```python
from build123d import *

# Parameters (mm, degrees)
F0_R     = 6.35
F1_DEPTH = 5.08
F2_SIZE  = 5.07999


# Not quite as in the source:
# - a fillet or chamfer is up to 0.001 mm smaller than in the source, because OpenCascade refuses the exact size


with BuildPart() as f1:
    # F0 (on Top) → F1 (new body)
    with BuildSketch(Plane.XY):
        with BuildLine():
            ThreePointArc((-16.2956875, 7.1118892639), (-12.5723585695, 12.5723585695), (-7.1118892639, 16.2956875))
            ThreePointArc((-7.1118892639, 16.2956875), (-6.7408857543, 18.5233780558), (-5.6901704054, 20.5224393535))
            Line((-5.6901704054, 20.5224393535), (-34.321730181, 34.321730181))
            Line((-34.321730181, 34.321730181), (-20.5224393535, 5.6901704054))
            ThreePointArc((-20.5224393535, 5.6901704054), (-18.5233780558, 6.7408857543), (-16.2956875, 7.1118892639))
        make_face()
        with BuildLine():
            ThreePointArc((16.2956875, -7.1118892639), (9.144, 0), (16.2956875, 7.1118892639))
            ThreePointArc((16.2956875, 7.1118892639), (12.5723585695, 12.5723585695), (7.1118892639, 16.2956875))
            ThreePointArc((7.1118892639, 16.2956875), (7.1119723159, 16.2758438272), (7.112, 16.256))
            ThreePointArc((7.112, 16.256), (-0.0198438272, 9.1440276841), (-7.1118892639, 16.2956875))
            ThreePointArc((-7.1118892639, 16.2956875), (-12.5723585695, 12.5723585695), (-16.2956875, 7.1118892639))
            ThreePointArc((-16.2956875, 7.1118892639), (-11.2411078526, 5.042955557), (-9.144, 0))
            ThreePointArc((-9.144, 0), (-11.2411078526, -5.042955557), (-16.2956875, -7.1118892639))
            ThreePointArc((-16.2956875, -7.1118892639), (-12.5723585695, -12.5723585695), (-7.1118892639, -16.2956875))
            ThreePointArc((-7.1118892639, -16.2956875), (-0.0198438272, -9.1440276841), (7.112, -16.256))
            ThreePointArc((7.112, -16.256), (7.1119723159, -16.2758438272), (7.1118892639, -16.2956875))
            ThreePointArc((7.1118892639, -16.2956875), (12.5723585695, -12.5723585695), (16.2956875, -7.1118892639))
        make_face()
        Circle(F0_R, mode=Mode.SUBTRACT)
        with BuildLine():
            ThreePointArc((7.1118892639, 16.2956875), (12.5723585695, 12.5723585695), (16.2956875, 7.1118892639))
            ThreePointArc((16.2956875, 7.1118892639), (18.5233780558, 6.7408857543), (20.5224393535, 5.6901704054))
            Line((20.5224393535, 5.6901704054), (34.321730181, 34.321730181))
            Line((34.321730181, 34.321730181), (5.6901704054, 20.5224393535))
            ThreePointArc((5.6901704054, 20.5224393535), (6.7408857543, 18.5233780558), (7.1118892639, 16.2956875))
        make_face()
        with BuildLine():
            ThreePointArc((20.5224393535, -5.6901704054), (18.5233780558, -6.7408857543), (16.2956875, -7.1118892639))
            ThreePointArc((16.2956875, -7.1118892639), (12.5723585695, -12.5723585695), (7.1118892639, -16.2956875))
            ThreePointArc((7.1118892639, -16.2956875), (6.7408857543, -18.5233780558), (5.6901704054, -20.5224393535))
            Line((5.6901704054, -20.5224393535), (34.321730181, -34.321730181))
            Line((34.321730181, -34.321730181), (20.5224393535, -5.6901704054))
        make_face()
        with BuildLine():
            ThreePointArc((-5.6901704054, -20.5224393535), (-6.7408857543, -18.5233780558), (-7.1118892639, -16.2956875))
            ThreePointArc((-7.1118892639, -16.2956875), (-12.5723585695, -12.5723585695), (-16.2956875, -7.1118892639))
            ThreePointArc((-16.2956875, -7.1118892639), (-18.5233780558, -6.7408857543), (-20.5224393535, -5.6901704054))
            Line((-20.5224393535, -5.6901704054), (-34.321730181, -34.321730181))
            Line((-34.321730181, -34.321730181), (-5.6901704054, -20.5224393535))
        make_face()
    extrude(amount=F1_DEPTH)

    # F2 (size 5.08 in the source; OpenCascade refuses exactly that, so slightly less here)
    f2_edges = [f1.edges().sort_by_distance(p)[0] for p in [
        (-27.422085, 20.00595, 5.08),
        (-20.00595, 27.422085, 5.08),
        (20.00595, 27.422085, 5.08),
        (27.422085, 20.00595, 5.08),
        (27.422085, -20.00595, 5.08),
        (20.00595, -27.422085, 5.08),
        (-20.00595, -27.422085, 5.08),
        (-27.422085, -20.00595, 5.08),
    ]]
    chamfer(f2_edges, length=F2_SIZE)


solid = f1.part
```
Geometry: final body of the model. Coordinates: model frame, mm. A direction names the side the tool comes from. Coordinates: 2 decimals unless noted, no trailing zeros. Order: outer loops, then holes, each group sorted by start corner. A loop starts at its lowest first (then second) coordinate and runs counter-clockwise, first axis right, second up. Notation, with made-up numbers: (-0.75, 42.5) - (20.25, 42.5) arc R15 ccw to (20.25, 53.5) - close; hole circle Ø9 at (-14, 69). An arc over 180 degrees is marked (long way). Return JSON: item names as keys, results as strings. Group by question number.
1. Cut plane D-D (y = 3). Output: boundary loops of the cut face in (x, z).
2. Set-up query: faces 1 (the face through (23.228, 17.236, 2.576)), 2 (the face through (-17.649, -23.427, 2.576)), 3 (the face through (-17.236, 23.228, 2.576)), 4 (the face through (-23.228, -17.236, 2.576)). Return all of +Z, -Z, +X, -X, +Y, -Y with unobstructed straight access to the full face (end or side cutting, diameter ignored); none if empty.
3. Pin query (flat end, axial travel): pin 1 (2 mm diameter, centred on x = 5.5, z = 2, fed in from +Y); pin 2 (1.5 mm diameter, centred on x = -13, z = 3.5, fed in from +Y); pin 3 (7.5 mm diameter, centred on x = 0, y = 0, fed in from +Z); pin 4 (1 mm diameter, centred on x = 22, z = 2.5, fed in from -Y). Return the tip coordinate at first contact, or that it passes through.
4. Cut plane A-A (x = 0). Output: boundary loops of the cut face in (y, z).
5. Pull-direction query (Y, two-part tool) for faces 5 (the face through (23.427, -17.649, 2.576)), 6 (the face through (17.649, 23.427, 2.576)), 7 (the face through (17.236, -23.228, 2.576)), 8 (the face through (0, 8, 0)); classes: pulls with the +Y half, pulls with the -Y half, needs draft (parallel to the pull), parting line crosses it, or undercut.
6. Material intervals for line 1 along Y through (x, z) = (0, 1.7); line 2 along X through (y, z) = (26, 3.4); line 3 along Y through (x, z) = (25, 2), sorted ascending. Write a range as [from, to].
Resolved:
{
 "1": {"outline": "(-9.81, 0) - (-5.6, 0) - (-5.6, 5.08) - (-9.81, 5.08) - close; (5.6, 0) - (9.81, 0) - (9.81, 5.08) - (5.6, 5.08) - close"},
 "2": {"face 1": "+Z, +X", "face 2": "+Z, -Y", "face 3": "+Z, +Y", "face 4": "+Z, -X"},
 "3": {"pin 1": "stops at y = 13.37", "pin 2": "stops at y = 21.07", "pin 3": "passes through", "pin 4": "stops at y = -26.21"},
 "4": {"outline": "(-9.14, 0) - (-6.35, 0) - (-6.35, 5.08) - (-9.14, 5.08) - close; (6.35, 0) - (9.14, 0) - (9.14, 5.08) - (6.35, 5.08) - close"},
 "5": {"face 5": "undercut", "face 6": "pulls with the +Y half", "face 7": "pulls with the -Y half", "face 8": "needs draft"},
 "6": {"line 1": "y = [-9.14, -6.35], [6.35, 9.14]", "line 2": "x = [-26.54, -24.89], [24.89, 26.54]", "line 3": "y = [-27.61, -19.59], [19.59, 27.61]"}
}
